from build123d import *

# Parameters (mm, degrees)
F1_DEPTH = 73.5
F2_W     = 70.3
F2_H     = 70.3
F3_DEPTH = 23
F4_DEPTH = 73.501


# Not quite as in the source:
# - a fillet or chamfer that OpenCascade refuses, or shapes differently, is made with other operations: its cross-section is extruded or revolved along the edge and cut away or added


with BuildPart() as f1:
    # F0 (on Front) → F1 (new body)
    with BuildSketch(Plane.XZ):
        with BuildLine():
            Line((0, 15), (0, 0))
            Line((0, 0), (73.5, 0))
            Line((73.5, 0), (73.5, 15))
            Line((73.5, 15), (46.75, 15))
            Line((46.75, 15), (38.75, 15))
            ThreePointArc((38.75, 15), (36.75, 13), (34.75, 15))
            Line((34.75, 15), (26.75, 15))
            Line((26.75, 15), (0, 15))
        make_face()
        with BuildLine():
            Line((0, 25), (0, 15))
            Line((0, 15), (26.75, 15))
            ThreePointArc((26.75, 15), (29.6789321881, 22.0710678119), (36.75, 25))
            Line((36.75, 25), (0, 25))
        make_face()
        with BuildLine():
            Line((46.75, 15), (73.5, 15))
            Line((73.5, 15), (73.5, 25))
            Line((73.5, 25), (36.75, 25))
            ThreePointArc((36.75, 25), (43.8210678119, 22.0710678119), (46.75, 15))
        make_face()
        with BuildLine():
            ThreePointArc((36.75, 25), (29.6789321881, 22.0710678119), (26.75, 15))
            Line((26.75, 15), (34.75, 15))
            ThreePointArc((34.75, 15), (36.75, 17), (38.75, 15))
            Line((38.75, 15), (46.75, 15))
            ThreePointArc((46.75, 15), (43.8210678119, 22.0710678119), (36.75, 25))
        make_face()
    extrude(amount=-F1_DEPTH)

    # F2 (on face) → F3 (cut)
    with BuildSketch(Plane.XY.offset(25)):
        with Locations((36.75, 36.75)):
            Rectangle(F2_W, F2_H)
    extrude(amount=-F3_DEPTH, mode=Mode.SUBTRACT)

    # F0 (on Front) → F4 (cut, through all)
    with BuildSketch(Plane.XZ):
        with BuildLine():
            Line((0, 25), (0, 15))
            Line((0, 15), (26.75, 15))
            ThreePointArc((26.75, 15), (29.6789321881, 22.0710678119), (36.75, 25))
            Line((36.75, 25), (0, 25))
        make_face()
        with BuildLine():
            Line((46.75, 15), (73.5, 15))
            Line((73.5, 15), (73.5, 25))
            Line((73.5, 25), (36.75, 25))
            ThreePointArc((36.75, 25), (43.8210678119, 22.0710678119), (46.75, 15))
        make_face()
    extrude(amount=-F4_DEPTH, mode=Mode.SUBTRACT)

    # F5: chamfer of 3 x 2 on 1 edges, made by hand

    # F5_s1 → F5_t2 (revolve, cut)
    with BuildSketch(Plane.XY.offset(15)):
        Polygon((34.75, 3), (32.75, 0), (34.75, 0), align=None)
    revolve(axis=Axis((36.75, 0, 15), (0, 1, 0)), mode=Mode.SUBTRACT)

    # F6: chamfer of 3 x 2 on 1 edges, made by hand

    # F6_s1 → F6_t2 (revolve, cut)
    with BuildSketch(Plane.XY.offset(15)):
        Polygon((32.75, 73.5), (34.75, 70.5), (34.75, 73.5), align=None)
    revolve(axis=Axis((36.75, 73.5, 15), (0, 1, 0)), mode=Mode.SUBTRACT)


solid = f1.part
The model under review builds one solid part; all positions refer to its coordinate system, in mm. A direction names the side the tool comes from. Give positions to 0.01 mm unless a question says otherwise; leave off trailing zeros. Order: outer loops, then holes, each group sorted by start corner. A loop starts at its lowest first (then second) coordinate and runs counter-clockwise, first axis right, second up. Notation, with made-up numbers: M 23,73 L 72,73 A25 ccw 72,86 Z; hole C -34.5,-34.75 d11. An arc over 180 degrees is marked long. Answer in a Markdown table with one row per item. Add a question column.
1. Add section A-A on z = 9. State the section outline as (x, y) points, plus the area to 3 significant figures.
2. Mouldability with a two-part tool opening along Z and no side actions: class faces 4 (the flat face through (36, 37, 2)), 5 (the flat face through (1.6, 36, 9)), 6 (the flat face through (36, 36, 0)) as released by +Z, released by -Z, zero draft, split by the parting line, or undercut.
3. Machinability: for faces 1 (the flat face through (1, 37, 15)), 2 (the flat face through (36, 1.6, 11)), 3 (the flat face through (73, 37, 15)), which of the approach directions +Z, -Z, +X, -X, +Y, -Y give a long, thin tool a straight path to every point of the face, cutting with its end or side? Answer none if there is none.
4. To check wall thickness, follow line 1 along Y through (x, z) = (41, 18); line 2 along Z through (x, y) = (68, 32.5). State the ranges of each line that lie inside material, in increasing order.
5. Add section B-B on y = 5. State the section outline as (x, z) points, plus the area to 3 significant figures.
6. Add section D-D on z = 23.25. State the section outline as (x, y) points.
7. For pin 1 Ø7 at (x, z) = (35, 9) entering from -Y; pin 2 Ø5 at (x, y) = (37, 65) entering from +Z; pin 3 Ø5 at (x, z) = (50, 21) entering from +Y, all flat-tipped, find the tip position at first contact; note any pin that passes through.
The answers:
| question | item | result |
|---|---|---|
| 1 | outline | M 0,0 L 73.5,0 L 73.5,73.5 L 0,73.5 Z; hole M 1.6,1.6 L 71.9,1.6 L 71.9,71.9 L 1.6,71.9 Z |
| 1 | area | 460 mm2 |
| 2 | face 4 | released by +Z |
| 2 | face 5 | zero draft |
| 2 | face 6 | released by -Z |
| 3 | face 1 | +Z, -X, +Y, -Y |
| 3 | face 2 | +Z |
| 3 | face 3 | +Z, +X, +Y, -Y |
| 4 | line 1 | 0 to 1.6, 71.9 to 73.5 |
| 4 | line 2 | 0 to 2 |
| 5 | outline | M 0,0 L 73.5,0 L 73.5,15 L 71.9,15 L 71.9,2 L 1.6,2 L 1.6,15 L 0,15 Z |
| 5 | area | 189 mm2 |
| 6 | outline | M 31.1,0 L 42.4,0 L 42.4,1.6 L 31.1,1.6 Z; M 31.1,71.9 L 42.4,71.9 L 42.4,73.5 L 31.1,73.5 Z |
| 7 | pin 1 | y = 0 |
| 7 | pin 2 | z = 2 |
| 7 | pin 3 | through |
